Input: dimensioned drawing with shaded views. Units: mm. Origin: part minimum x, y, z. A direction names the side the tool comes from. Round coordinates to 2 decimals unless told otherwise and drop trailing zeros. Order: outer loops, then holes, each group sorted by start corner. A loop starts at its lowest first (then second) coordinate and runs counter-clockwise, first axis right, second up. Notation, with made-up numbers: (60, -24.75) -> (73, -24.75) arc R19 ccw to (73, 2.25) -> close; hole circle Ø4 at (17, 54). An arc over 180 degrees is marked (long way). Use a Markdown table: item, result. Add a question column.
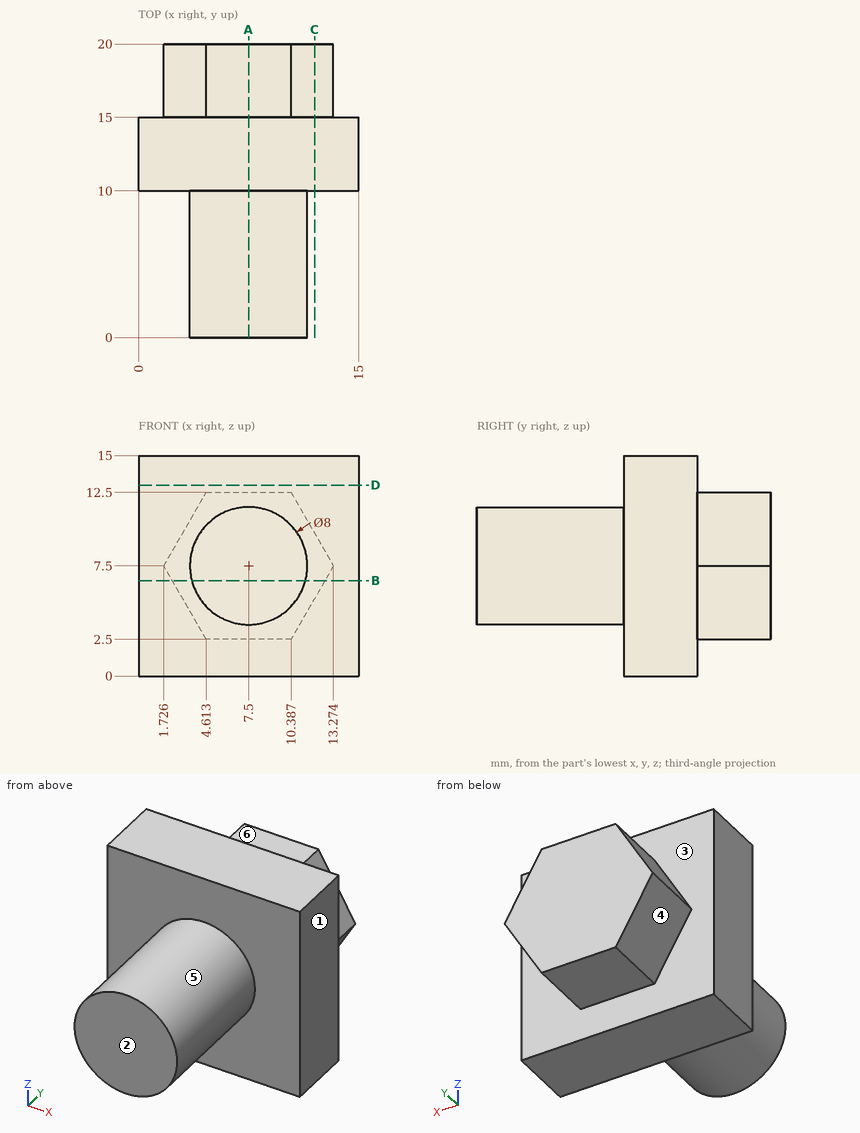
1) Reachability of the marked faces 4, 5 and 6 from +Z, -Z, +X, -X, +Y, -Y: full face, straight path, thin tool, end or side. Return the list, or none.
2) First-contact query: pin 1 Ø2 at (x, y) = (8, 4.5) entering from -Z; pin 2 Ø2.5 at (x, y) = (7, 17) entering from -Z; pin 3 Ø5.5 at (x, y) = (7, 18) entering from +Z. Flat tips, straight axial feed; report the tip coordinate or a pass-through.
3) Section A-A on x = 7.5. Output: boundary loops of the cut face in (y, z).
4) Section D-D on z = 13. Output: boundary loops of the cut face in (x, y).
5) Section B-B on z = 6.5. Output: boundary loops of the cut face in (x, y), then the cut area to 3 significant figures.
6) Draft query along Y for the marked faces 1, 2 and 3. Return one class per face: pulls with the +Y half, pulls with the -Y half, needs draft (parallel to the pull), parting line crosses it, or undercut.
7) Line query: probe 1 along Y at (x, z) = (2.5, 9); probe 2 along Y at (x, z) = (3.5, 10); probe 3 along Z at (x, y) = (6.25, 7.75). Output: solid intervals per line, ascending. Write a range as from..to.
8) Section C-C on x = 12. Output: boundary loops of the cut face in (y, z) (1 decimal).
Conclusion:
| question | item | result |
|---|---|---|
| 1 | face 4 | -Z, -X, +Y |
| 1 | face 5 | -Y |
| 1 | face 6 | +Z, +X, -X, +Y |
| 2 | pin 1 | stops at z = 3.5 |
| 2 | pin 2 | stops at z = 2.5 |
| 2 | pin 3 | stops at z = 12.5 |
| 3 | outline | (0, 3.5) -> (10, 3.5) -> (10, 0) -> (15, 0) -> (15, 2.5) -> (20, 2.5) -> (20, 12.5) -> (15, 12.5) -> (15, 15) -> (10, 15) -> (10, 11.5) -> (0, 11.5) -> close |
| 4 | outline | (0, 10) -> (15, 10) -> (15, 15) -> (0, 15) -> close |
| 5 | outline | (0, 10) -> (3.63, 10) -> (3.63, 0) -> (11.37, 0) -> (11.37, 10) -> (15, 10) -> (15, 15) -> (12.7, 15) -> (12.7, 20) -> (2.3, 20) -> (2.3, 15) -> (0, 15) -> close |
| 5 | area | 204 mm^2 |
| 6 | face 1 | needs draft |
| 6 | face 2 | pulls with the -Y half |
| 6 | face 3 | pulls with the +Y half |
| 7 | probe 1 | y = 10..15 |
| 7 | probe 2 | y = 10..20 |
| 7 | probe 3 | z = 3.7..11.3 |
| 8 | outline | (10, 0) -> (15, 0) -> (15, 5.3) -> (20, 5.3) -> (20, 9.7) -> (15, 9.7) -> (15, 15) -> (10, 15) -> close |
